from build123d import *

# Parameters (mm, degrees)
SKETCH1_W           = 200
SKETCH1_H           = 50
BOSS_EXTRUDE1_DEPTH = 40
SKETCH2_R           = 6.35
CUT_EXTRUDE1_DEPTH  = 111.566721937
SKETCH4_W           = 20
SKETCH4_H           = 40
CUT_EXTRUDE2_DEPTH  = 206.48722588


with BuildPart() as part:
    # Sketch1 → Boss-Extrude1 (new body)
    with BuildSketch(Plane.XY):
        Rectangle(SKETCH1_W, SKETCH1_H)
    extrude(amount=BOSS_EXTRUDE1_DEPTH)

    # Sketch2 → Cut-Extrude1 (cut, through all)
    with BuildSketch(Plane.XY.offset(40)):
        with Locations((90, 15)):
            Circle(SKETCH2_R)
        with Locations((46.75, 15)):
            Circle(SKETCH2_R)
    extrude(amount=-CUT_EXTRUDE1_DEPTH, mode=Mode.SUBTRACT)

    # Sketch4 → Cut-Extrude2 (cut, through all)
    with BuildSketch(Plane.ZY.offset(100)):
        with Locations((20, 5)):
            Rectangle(SKETCH4_W, SKETCH4_H)
    extrude(amount=-CUT_EXTRUDE2_DEPTH, mode=Mode.SUBTRACT)


solid = part.part
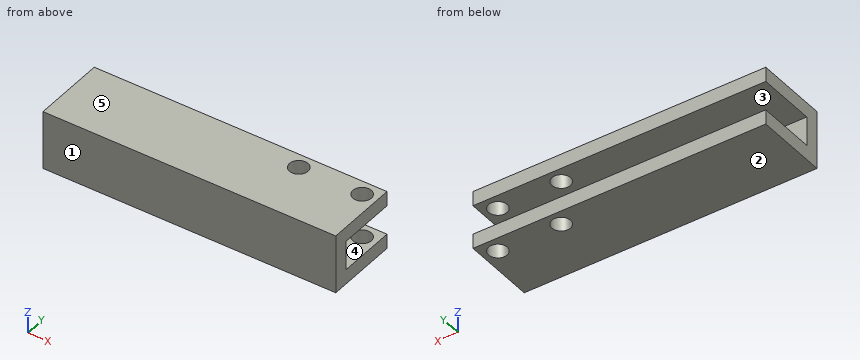
Model file for the job. Use its own axes, mm. Face numbers are marked on the shaded views. A direction names the side the tool comes from. Give positions to 0.01 mm unless a question says otherwise; leave off trailing zeros. Loops run counter-clockwise (first coordinate to the right, second up) from the corner with the lowest first, then second, coordinate; pieces in that order, holes last. Notation, with made-up numbers: (30, 11.25) -> (35, 11.25) arc R17 cw to (35, 28.25) -> close; hole circle Ø7 at (36.25, 33.5). An arc over 180 degrees is marked (long way). Use a Markdown table: item, result. Add a question column.
(1) Wall check: line 1 along Z through (x, y) = (28, 13); line 2 along Y through (x, z) = (90, 4); line 3 along X through (y, z) = (20.5, 35). Give the ranges that are in metal, low to high.
(2) Slice it at C-C on x = 46.75. List the corners of the cut face in (y, z).
(3) Slice it at B-B on y = 0. List the corners of the cut face in (x, z), and give its area (3 significant figures).
(4) Slice it at A-A on y = 15. List the corners of the cut face in (x, z), and give its area (3 significant figures).
(5) Tool access for the marked faces 4 and 5: list every direction of +Z, -Z, +X, -X, +Y, -Y with a clear straight run to the whole face (end or side of a thin tool).
(6) Slice it at D-D on x = 77. List the corners of the cut face in (y, z).
(7) Drop a flat-ended pin along its axis: pin 1 Ø16.5 at (x, y) = (46.75, 15) entering from +Z. Give the stop position or say it passes through.
(8) Mould opens along Z. For the marked faces 1, 2 and 3 say: +Z half, -Z half, draft (parallel to the pull), parting line (faces both ways), or undercut.
Filled sheet:
| question | item | result |
|---|---|---|
| 1 | line 1 | 0 to 10, 30 to 40 |
| 1 | line 2 | -25 to 8.65, 21.35 to 25 |
| 1 | line 3 | -100 to 43.58, 49.92 to 86.83, 93.17 to 100 |
| 2 | outline | (-25, 0) -> (8.65, 0) -> (8.65, 10) -> (-15, 10) -> (-15, 30) -> (8.65, 30) -> (8.65, 40) -> (-25, 40) -> close; (21.35, 0) -> (25, 0) -> (25, 10) -> (21.35, 10) -> close; (21.35, 30) -> (25, 30) -> (25, 40) -> (21.35, 40) -> close |
| 3 | outline | (-100, 0) -> (100, 0) -> (100, 10) -> (-100, 10) -> close; (-100, 30) -> (100, 30) -> (100, 40) -> (-100, 40) -> close |
| 3 | area | 4,000 mm2 |
| 4 | outline | (-100, 0) -> (40.4, 0) -> (40.4, 10) -> (-100, 10) -> close; (-100, 30) -> (40.4, 30) -> (40.4, 40) -> (-100, 40) -> close; (53.1, 0) -> (83.65, 0) -> (83.65, 10) -> (53.1, 10) -> close; (53.1, 30) -> (83.65, 30) -> (83.65, 40) -> (53.1, 40) -> close; (96.35, 0) -> (100, 0) -> (100, 10) -> (96.35, 10) -> close; (96.35, 30) -> (100, 30) -> (100, 40) -> (96.35, 40) -> close |
| 4 | area | 3,490 mm2 |
| 5 | face 4 | +X, -X, +Y |
| 5 | face 5 | +Z, +X, -X, +Y, -Y |
| 6 | outline | (-25, 0) -> (25, 0) -> (25, 10) -> (-15, 10) -> (-15, 30) -> (25, 30) -> (25, 40) -> (-25, 40) -> close |
| 7 | pin 1 | z = 40 |
| 8 | face 1 | draft |
| 8 | face 2 | -Z half |
| 8 | face 3 | undercut |
